```python
from build123d import *

# Parameters (mm, degrees)
SKETCH1_R                = 1.5
BOSS_EXTRUDE1_DEPTH      = 2
FILLET1_R                = 6
FILLET2_R                = 3
F_3_0_3_DIAMETER_HOLE1_D = 3


with BuildPart() as part:
    # Sketch1 → Boss-Extrude1 (new body)
    with BuildSketch(Plane(origin=(0, 0, 0), x_dir=(1, 0, 0), z_dir=(0, 1, 0))):
        with BuildLine():
            Line((-74.629040009, 40.687914512), (-63.639610307, 29.69848481))
            Line((-63.639610307, 29.69848481), (-42.426406871, 50.911688245))
            Line((-42.426406871, 50.911688245), (-36.769552622, 45.254833996))
            Line((-36.769552622, 45.254833996), (-68.72500623, 13.299380388))
            ThreePointArc((-68.72500623, 13.299380388), (-69.616532676, 7.316992429), (-69.988296617, 1.279975229))
            Line((-69.988296617, 1.279975229), (-45.375058731, -36.621087439))
            Line((-45.375058731, -36.621087439), (-52.084423274, -40.978199719))
            Line((-52.084423274, -40.978199719), (-68.423594325, -15.81808268))
            Line((-68.423594325, -15.81808268), (-81.457709532, -24.282536066))
            ThreePointArc((-81.457709532, -24.282536066), (-84.534361106, 8.884919378), (-74.629040009, 40.687914512))
        make_face()
        with Locations((-43.840620434, 43.840620434)):
            Circle(SKETCH1_R, mode=Mode.SUBTRACT)
        with Locations((-59.39696962, 28.284271247)):
            Circle(SKETCH1_R, mode=Mode.SUBTRACT)
        with Locations((-51.997575213, -33.767620171)):
            Circle(SKETCH1_R, mode=Mode.SUBTRACT)
        with Locations((-63.979633983, -15.316867676)):
            Circle(SKETCH1_R, mode=Mode.SUBTRACT)
    extrude(amount=BOSS_EXTRUDE1_DEPTH)

    # Fillet1
    fillet1_edges = [part.edges().sort_by_distance(p)[0] for p in [
        (-74.629040009, 1, -40.687914512),
        (-81.457709532, 1, 24.282536066),
    ]]
    fillet(fillet1_edges, radius=FILLET1_R)

    # Fillet2
    fillet2_edges = [part.edges().sort_by_distance(p)[0] for p in [
        (-63.639610307, 1, -29.69848481),
        (-68.72500623, 1, -13.299380388),
        (-69.988296617, 1, -1.279975229),
        (-68.423594325, 1, 15.81808268),
    ]]
    fillet(fillet2_edges, radius=FILLET2_R)

    # Ø3.0 (3) Diameter Hole1 (through all)
    with Locations(Plane(origin=(0, 2, 0), x_dir=(1, 0, 0), z_dir=(0, 1, 0))):
        with Locations((-80.534361106, 8.884919378)):
            Hole(F_3_0_3_DIAMETER_HOLE1_D / 2)


solid = part.part
```
Check sheet for the modelled part. Datum: model origin and axes. Units: mm. A direction names the side the tool comes from. Coordinates: 2 decimals unless noted, no trailing zeros. Loops run counter-clockwise (first coordinate to the right, second up) from the corner with the lowest first, then second, coordinate; pieces in that order, holes last.
1) Sectioned sample at B-B (y = 1.35). Record the boundary of the cut face in (x, z).
2) Release check for a two-part mould opening along X. For faces 1 (the face through (-73.97, 1.014, -36.366)), 2 (the face through (-68.714, 1.014, 17.027)), 3 (the face through (-84.57, 0.99, -8.54)), 4 (the face through (-69.86, 1.01, -1.34)) record: released by +X, released by -X, zero draft, split by the parting line, or undercut.
3) Sectioned sample at A-A (x = -54.5). Record the boundary of the cut face in (y, z), and give its area (3 significant figures).
4) Access from +Z, -Z, +X, -X, +Y, -Y to the whole of each face (thin tool, end or side, straight path). Record for faces 5 (the face through (-67.22, 0.99, -33.28)), 6 (the face through (-70, 2, -9)), 7 (the face through (-68.599, 1.014, -13.236)).
5) Material ranges on probe 1 along Z at (x, y) = (-52.5, 1); probe 2 along Z at (x, y) = (-51, 1); probe 3 along Z at (x, y) = (-67, 0.65), recorded low to high.
6) Sectioned sample at D-D (z = -17). Record the boundary of the cut face in (x, y), and give its area (3 significant figures).
7) Sectioned sample at C-C (x = -49). Record the boundary of the cut face in (y, z).
8) Gauge pin test, flat end, axial feed: pin 1 (5 mm diameter, centred on x = -59.4, z = -28.28, fed in from +Y). Record the tip position at first contact, or that the pin passes through.
Check sheet entries:
1. outline: (-83.53, 15.76) arc R85 ccw to (-78.43, -32.78) arc R6 ccw to (-68.65, -34.71) - (-65.76, -31.82) arc R3 cw to (-61.52, -31.82) - (-42.43, -50.91) - (-36.77, -45.25) - (-68.07, -13.96) arc R3 cw to (-68.9, -12.37) arc R70 cw to (-69.96, -2.23) arc R3 cw to (-69.48, -0.5) - (-45.38, 36.62) - (-52.08, 40.98) - (-66.79, 18.33) arc R3 cw to (-70.94, 17.45) - (-74.36, 19.68) arc R6 ccw to start; hole circle Ø3 at (-80.53, -8.88); hole circle Ø3 at (-63.98, 15.32); hole circle Ø3 at (-59.4, -28.28); hole circle Ø3 at (-52, 33.77); hole circle Ø3 at (-43.84, -43.84)
2. face 1: undercut
2. face 2: undercut
2. face 3: released by -X
2. face 4: released by +X
3. outline: (0, -38.84) - (2, -38.84) - (2, -27.52) - (0, -27.52) - close; (0, 22.57) - (2, 22.57) - (2, 37.26) - (0, 37.26) - close
3. area: 52.0 mm2
4. face 5: -Z, +Y, -Y
4. face 6: +Z, -Z, +X, -X, +Y
4. face 7: +X, +Y, -Y
5. probe 1: z = -40.84 to -29.52, 25.65 to 32.35, 35.18 to 40.34
5. probe 2: z = -42.34 to -31.02, 27.96 to 32.65, 34.89 to 40.27
5. probe 3: z = -33.06 to -15.02, 3.32 to 18.05
6. outline: (-83.28, 0) - (-65.02, 0) - (-65.02, 2) - (-83.28, 2) - close
6. area: 36.5 mm2
7. outline: (0, -44.34) - (2, -44.34) - (2, -33.02) - (0, -33.02) - close; (0, 31.04) - (2, 31.04) - (2, 38.98) - (0, 38.98) - close
8. pin 1: stops at y = 2
